For this review, use the dimensioned drawing (mm, ordinates from the lowest corner) and the shaded views. Round coordinates to 2 decimals unless told otherwise and drop trailing zeros. Loops run counter-clockwise (first coordinate to the right, second up) from the corner with the lowest first, then second, coordinate; pieces in that order, holes last.
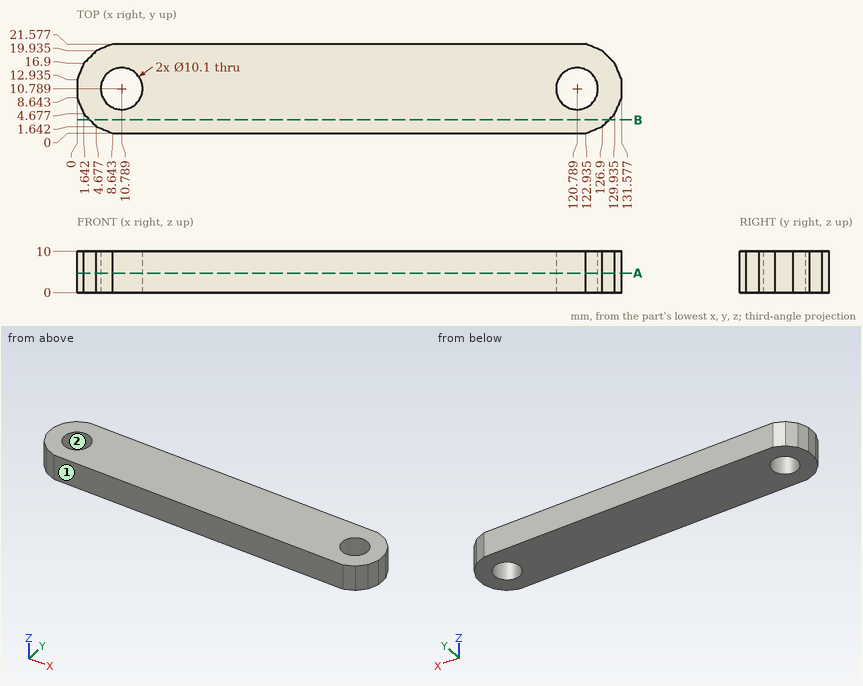
(1) Add section B-B (y = 3.25). Give the boundary of the cut face in (x, z), plus the area to 3 significant figures.
(2) For L1, parallel to X at y = 6.5, z = 7.75 (1 decimal); L2, parallel to X at y = 7.25, z = 3 (1 decimal); L3, parallel to Y at x = 12, z = 5.75 (1 decimal), list the stretches that pass through material, from the lowest coordinate up.
(3) The part is to be moulded in two halves that separate along X. For the marked faces 1 and 2, say which applies: pulls with the +X half, pulls with the -X half, needs draft (parallel to the pull), parting line crosses it, or undercut.
(4) Add section A-A (z = 4.75). Give the number of separate pieces and of enclosed holes in the cut face, plus the area to 3 significant figures.
Outcome:
1. outline: (3.07, 0) - (128.51, 0) - (128.51, 10) - (3.07, 10) - close
1. area: 1,250 mm2
2. L1: x = 0.9 to 8.1, 13.5 to 118.1, 123.5 to 130.7
2. L2: x = 0.6 to 7.2, 14.4 to 117.2, 124.4 to 131
2. L3: y = 0 to 5.9, 15.7 to 21.6
3. face 1: needs draft
3. face 2: undercut
4. separate pieces: 1
4. enclosed holes: 2
4. area: 2,580 mm2
